```python
from build123d import *

# Parameters (mm, degrees)
BOSS_EXTRUDE1_DEPTH      = 6
CUT_EXTRUDE1_DEPTH       = 6
M5_CLEARANCE_HOLE1_D     = 5.5
CUT_EXTRUDE2_DEPTH       = 22
M5_CLEARANCE_HOLE2_D     = 5.5
CUT_EXTRUDE3_DEPTH       = 6
CUT_EXTRUDE4_DEPTH       = 6
M3_CLEARANCE_HOLE1_D     = 3.4
M3_CLEARANCE_HOLE1_DEPTH = 10
M3_CLEARANCE_HOLE1_TIP   = 1.021463052


with BuildPart() as part:
    # Sketch2 → Boss-Extrude1 (new body)
    with BuildSketch(Plane.XY):
        with BuildLine():
            Line((-55, -80), (55, -80))
            ThreePointArc((55, -80), (58.535533906, -78.535533906), (60, -75))
            Line((60, -75), (60, 75))
            ThreePointArc((60, 75), (58.535533906, 78.535533906), (55, 80))
            Line((55, 80), (-55, 80))
            ThreePointArc((-55, 80), (-58.535533906, 78.535533906), (-60, 75))
            Line((-60, 75), (-60, -75))
            ThreePointArc((-60, -75), (-58.535533906, -78.535533906), (-55, -80))
        make_face()
    extrude(amount=BOSS_EXTRUDE1_DEPTH)

    # Sketch3 → Cut-Extrude1 (cut)
    with BuildSketch(Plane.XY.offset(6)):
        with BuildLine():
            Line((2.75, -17.5), (2.75, -62.5))
            ThreePointArc((2.75, -62.5), (0, -65.25), (-2.75, -62.5))
            Line((-2.75, -62.5), (-2.75, -17.5))
            ThreePointArc((-2.75, -17.5), (0, -14.75), (2.75, -17.5))
        make_face()
    extrude(amount=-CUT_EXTRUDE1_DEPTH, mode=Mode.SUBTRACT)

    # M5 Clearance Hole1 (through all)
    with Locations(Plane.XY.offset(6)):
        with Locations((-23.57, -63.57), (-23.57, -16.43), (23.57, -16.43), (23.57, -63.57)):
            Hole(M5_CLEARANCE_HOLE1_D / 2)

    # Sketch6 → Cut-Extrude2 (cut)
    with BuildSketch(Plane.XY.offset(6)):
        with BuildLine():
            Line((-31.82, -16.43), (-31.82, -23.43))
            ThreePointArc((-31.82, -23.43), (-34.57, -26.18), (-37.32, -23.43))
            Line((-37.32, -23.43), (-37.32, -16.43))
            ThreePointArc((-37.32, -16.43), (-34.57, -13.68), (-31.82, -16.43))
        make_face()
    cut_extrude2 = extrude(amount=-CUT_EXTRUDE2_DEPTH, mode=Mode.SUBTRACT)

    # M5 Clearance Hole2 (through all)
    with Locations(Plane.XY.offset(6)):
        with Locations((-34.57, 41.47)):
            m5_clearance_hole2 = Hole(M5_CLEARANCE_HOLE2_D / 2)

    # Sketch9 → Cut-Extrude3 (cut)
    with BuildSketch(Plane.XY.offset(6)):
        with BuildLine():
            Line((-46.82, 25.07), (-46.82, -64.93))
            ThreePointArc((-46.82, -64.93), (-49.57, -67.68), (-52.32, -64.93))
            Line((-52.32, -64.93), (-52.32, 25.07))
            ThreePointArc((-52.32, 25.07), (-49.57, 27.82), (-46.82, 25.07))
        make_face()
    cut_extrude3 = extrude(amount=-CUT_EXTRUDE3_DEPTH, mode=Mode.SUBTRACT)

    # Mirror2: Cut-Extrude2, M5 Clearance Hole2, Cut-Extrude3 across plane
    add(cut_extrude2.mirror(Plane(origin=(0, 0, 0), x_dir=(0, 0, 1), z_dir=(1, 0, 0))), mode=Mode.SUBTRACT)
    add(m5_clearance_hole2.mirror(Plane(origin=(0, 0, 0), x_dir=(0, 0, 1), z_dir=(1, 0, 0))), mode=Mode.SUBTRACT)
    add(cut_extrude3.mirror(Plane(origin=(0, 0, 0), x_dir=(0, 0, 1), z_dir=(1, 0, 0))), mode=Mode.SUBTRACT)

    # Sketch11 → Cut-Extrude4 (cut)
    with BuildSketch(Plane.XY.offset(6)):
        with BuildLine():
            Line((-7.25, 68.5), (-7.25, 61.5))
            ThreePointArc((-7.25, 61.5), (-10, 58.75), (-12.75, 61.5))
            Line((-12.75, 61.5), (-12.75, 68.5))
            ThreePointArc((-12.75, 68.5), (-10, 71.25), (-7.25, 68.5))
        make_face()
        with BuildLine():
            Line((12.75, 68.5), (12.75, 61.5))
            ThreePointArc((12.75, 61.5), (10, 58.75), (7.25, 61.5))
            Line((7.25, 61.5), (7.25, 68.5))
            ThreePointArc((7.25, 68.5), (10, 71.25), (12.75, 68.5))
        make_face()
    extrude(amount=-CUT_EXTRUDE4_DEPTH, mode=Mode.SUBTRACT)

    # M3 Clearance Hole1
    with Locations(Plane.XY.offset(6)):
        with Locations((-7, -34), (7, -34), (7, -70), (-7, -70)):
            Hole(M3_CLEARANCE_HOLE1_D / 2, depth=M3_CLEARANCE_HOLE1_DEPTH)
            with Locations((0, 0, -(M3_CLEARANCE_HOLE1_DEPTH + M3_CLEARANCE_HOLE1_TIP / 2))):  # 118° drill point
                Cone(0, M3_CLEARANCE_HOLE1_D / 2, M3_CLEARANCE_HOLE1_TIP, mode=Mode.SUBTRACT)


solid = part.part
```
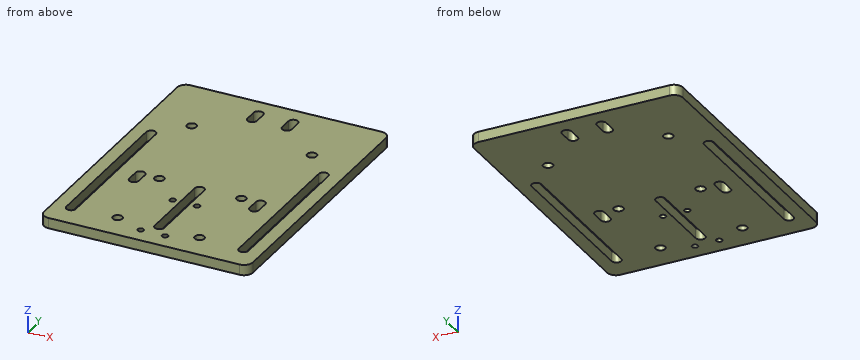
Model file for the job. Use its own axes, mm. Round coordinates to 2 decimals unless told otherwise and drop trailing zeros. Write each loop counter-clockwise with the first axis right and the second up, starting at its lowest first coordinate (ties: lowest second). Pieces come first, ordered by that corner, then holes. Notation, with made-up numbers: (-25.5, -33.5) - (23.5, -33.5) arc R20 ccw to (23.5, -22.5) - close; hole circle Ø9 at (18.5, -15). An arc over 180 degrees is marked (long way). One line per item, written item: value.
(1) Drop flat-ended pins along their axis: P1, Ø3.5, axis at x = 34.57, y = 41.47, coming from the -Z side; P2, Ø5.5, axis at x = 7, y = -34, coming from the +Z side. Give the stop position or say it passes through.
Values follow:
P1: passes through
P2: stops at z = 6
(2) Cut at A-A, the plane x = 49.57. Give the cut face in (y, z), plus the area to 3 significant figures.
Values follow:
outline: (-80, 0) - (-67.68, 0) - (-67.68, 6) - (-80, 6) - close; (27.82, 0) - (80, 0) - (80, 6) - (27.82, 6) - close
area: 387 mm²
(3) Cut at C-C, the plane y = -55. Give the cut face in (x, z).
Values follow:
outline: (-60, 0) - (-52.32, 0) - (-52.32, 6) - (-60, 6) - close; (-46.82, 0) - (-2.75, 0) - (-2.75, 6) - (-46.82, 6) - close; (2.75, 0) - (46.82, 0) - (46.82, 6) - (2.75, 6) - close; (52.32, 0) - (60, 0) - (60, 6) - (52.32, 6) - close
(4) Cut at B-B, the plane y = -7. Give the cut face in (x, z), plus the area to 3 significant figures.
Values follow:
outline: (-60, 0) - (-52.32, 0) - (-52.32, 6) - (-60, 6) - close; (-46.82, 0) - (46.82, 0) - (46.82, 6) - (-46.82, 6) - close; (52.32, 0) - (60, 0) - (60, 6) - (52.32, 6) - close
area: 654 mm²
(5) Cut at D-D, the plane x = 23.57. Give the cut face in (y, z).
Values follow:
outline: (-80, 0) - (-66.32, 0) - (-66.32, 6) - (-80, 6) - close; (-60.82, 0) - (-19.18, 0) - (-19.18, 6) - (-60.82, 6) - close; (-13.68, 0) - (80, 0) - (80, 6) - (-13.68, 6) - close
(6) Wall check: probe 1 along X at (y, z) = (-70, 2.2); probe 2 along X at (y, z) = (-54, 1.75); probe 3 along X at (y, z) = (18.5, 3.2). Give the ranges that are in metal, low to high.
Values follow:
probe 1: x = -60 to -8.7, -5.3 to 5.3, 8.7 to 60
probe 2: x = -60 to -52.32, -46.82 to -2.75, 2.75 to 46.82, 52.32 to 60
probe 3: x = -60 to -52.32, -46.82 to 46.82, 52.32 to 60
